from build123d import *

# Parameters (mm, degrees)
SKETCH1_W                 = 71.17230149
SKETCH1_H                 = 12.54
BOSS_EXTRUDE1_DEPTH       = 7.25
SHELL1_T                  = -0.5
SHELL1_THICKNESS_2_FACE_W = 70.17230149
SHELL1_THICKNESS_2_FACE_H = 11.54
SHELL1_THICKNESS_2_DEPTH  = 0.3


with BuildPart() as part:
    # Sketch1 → Boss-Extrude1 (new body)
    with BuildSketch(Plane.XY):
        with Locations((43.450650745, 55.8)):
            Rectangle(SKETCH1_W, SKETCH1_H)
    extrude(amount=BOSS_EXTRUDE1_DEPTH)

    # Shell1
    shell1_openings = [part.faces().sort_by_distance(p)[0] for p in [
        (43.450650745, 55.8, 0),
    ]]
    offset(amount=SHELL1_T, openings=shell1_openings, kind=Kind.INTERSECTION)

    # Shell1 thickness 2 face (on inner face of the shell) → Shell1 thickness 2 (cut)
    with BuildSketch(Plane(origin=(43.450650745, 55.8, 6.75), x_dir=(1, 0, 0), z_dir=(0, 0, 1))):
        Rectangle(SHELL1_THICKNESS_2_FACE_W, SHELL1_THICKNESS_2_FACE_H)
    extrude(amount=SHELL1_THICKNESS_2_DEPTH, mode=Mode.SUBTRACT)


solid = part.part
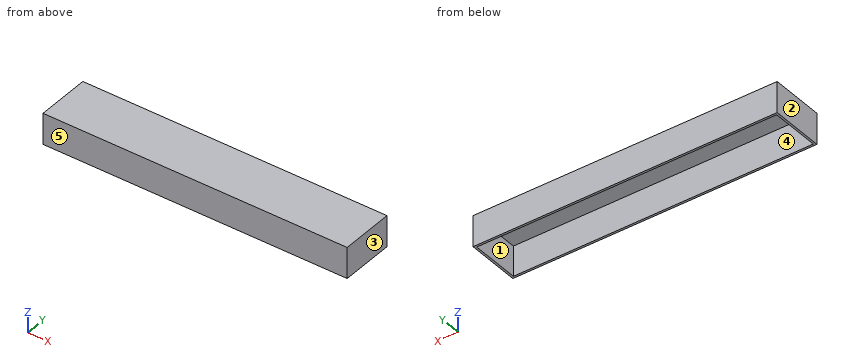
Read the model definition and answer for the solid it produces. Units are mm, in the model's axes. Face numbers are marked on the shaded views. A direction names the side the tool comes from. Round coordinates to 2 decimals unless told otherwise and drop trailing zeros. Order: outer loops, then holes, each group sorted by start corner. A loop starts at its lowest first (then second) coordinate and runs counter-clockwise, first axis right, second up.
1) A flat-ended cylindrical pin translates along its axis: pin 1 (6 mm diameter, centred on x = 40, y = 53.5, fed in from -Z). Find the tip coordinate at first contact, or state that the pin passes through.
2) The mould has two halves that part along X. Classify the marked faces 3, 4 and 5: released by +X, released by -X, zero draft, split by the parting line, or undercut.
3) The part is cut by section A-A on z = 5. Write down the section's boundary in (x, y), plus the area to 3 significant figures.
4) For the marked faces 1 and 2, determine the directions among +Z, -Z, +X, -X, +Y, -Y from which every point of the face is accessible in a straight line to the end or side of a thin tool.
5) The part is cut by section C-C on x = 15.5. Write down the section's boundary in (y, z), plus the area to 3 significant figures.
6) Straight lines are drawn through the part: L1, parallel to X at y = 59, z = 1.25; L2, parallel to Y at x = 19, z = 3.75; L3, parallel to Z at x = 39.5, y = 59. For each, find the intervals that lie inside material, in ascending order.
7) The part is cut by section B-B on y = 55.75. Write down the section's boundary in (x, z).
Resolved:
1. pin 1: stops at z = 7.05
2. face 3: released by +X
2. face 4: undercut
2. face 5: zero draft
3. outline: (7.86, 49.53) - (79.04, 49.53) - (79.04, 62.07) - (7.86, 62.07) - close; hole (8.36, 50.03) - (78.54, 50.03) - (78.54, 61.57) - (8.36, 61.57) - close
3. area: 82.7 mm2
4. face 1: -Z
4. face 2: +Z, -Z, -X, +Y, -Y
5. outline: (49.53, 0) - (50.03, 0) - (50.03, 7.05) - (61.57, 7.05) - (61.57, 0) - (62.07, 0) - (62.07, 7.25) - (49.53, 7.25) - close
5. area: 9.56 mm2
6. L1: x = 7.86 to 8.36, 78.54 to 79.04
6. L2: y = 49.53 to 50.03, 61.57 to 62.07
6. L3: z = 7.05 to 7.25
7. outline: (7.86, 0) - (8.36, 0) - (8.36, 7.05) - (78.54, 7.05) - (78.54, 0) - (79.04, 0) - (79.04, 7.25) - (7.86, 7.25) - close
